Design review of the part built by this model. Coordinates are the model's own, in mm. A direction names the side the tool comes from. Coordinates: 2 decimals unless noted, no trailing zeros. Write each loop counter-clockwise with the first axis right and the second up, starting at its lowest first coordinate (ties: lowest second). Pieces come first, ordered by that corner, then holes. Notation, with made-up numbers: (86, 38.25) - (104, 38.25) arc R19 ccw to (104, 69.25) - close; hole circle Ø11 at (-21.5, -8.75). An arc over 180 degrees is marked (long way). One line per item, written item: value.
from build123d import *

# Parameters (mm, degrees)
F1_DEPTH = 30


with BuildPart() as f1:
    # F0 (on Front) → F1 (new body)
    with BuildSketch(Plane.XZ):
        with BuildLine():
            Line((-10.025, -10.025), (-10.025, -4.563699))
            Line((-10.025, -4.563699), (-8.201301, -2.74))
            Line((-8.201301, -2.74), (-8.125, -2.74))
            Line((-8.125, -2.74), (-8.125, -4.16967))
            Line((-8.125, -4.16967), (-7.125, -4.16967))
            Line((-7.125, -4.16967), (-6.125, -2.504835))
            Line((-6.125, -2.504835), (-6.125, -0.84))
            Line((-6.125, -0.84), (-9.129728, -0.84))
            Line((-9.129728, -0.84), (-12.025, -3.735272))
            Line((-12.025, -3.735272), (-16.854638, -12.46486))
            ThreePointArc((-16.854638, -12.46486), (-17.38041, -18.730472), (-12.025, -22.025))
            Line((-12.025, -22.025), (12.025, -22.025))
            ThreePointArc((12.025, -22.025), (17.29087, -18.900868), (17.072982, -12.781872))
            Line((17.072982, -12.781872), (12.025, -3.735272))
            Line((12.025, -3.735272), (9.129728, -0.84))
            Line((9.129728, -0.84), (6.125, -0.84))
            Line((6.125, -0.84), (6.125, -2.504835))
            Line((6.125, -2.504835), (7.125, -4.16967))
            Line((7.125, -4.16967), (8.125, -4.16967))
            Line((8.125, -4.16967), (8.125, -2.74))
            Line((8.125, -2.74), (8.201301, -2.74))
            Line((8.201301, -2.74), (10.025, -4.563699))
            Line((10.025, -4.563699), (10.025, -10.025))
            Line((10.025, -10.025), (4.636716, -10.025))
            Line((4.636716, -10.025), (2.811716, -8.2))
            Line((2.811716, -8.2), (-2.811716, -8.2))
            Line((-2.811716, -8.2), (-4.636716, -10.025))
            Line((-4.636716, -10.025), (-8.125, -10.025))
            Line((-8.125, -10.025), (-10.025, -10.025))
        make_face()
        with BuildLine():
            ThreePointArc((-14.436503, -19.21634), (-15.81745, -14.753261), (-12.025, -12.025))
            Line((-12.025, -12.025), (-1.797092, -12.025))
            Line((-1.797092, -12.025), (-1.245732, -12.853762))
            Line((-1.245732, -12.853762), (-10.966173, -19.320583))
            ThreePointArc((-10.966173, -19.320583), (-12.71795, -19.821483), (-14.436503, -19.21634))
        make_face(mode=Mode.SUBTRACT)
        with BuildLine():
            Line((4.803493, -20.025), (-4.803493, -20.025))
            Line((-4.803493, -20.025), (-1.661703, -17.934828))
            ThreePointArc((-1.661703, -17.934828), (0, -17.432575), (1.661703, -17.934828))
            Line((1.661703, -17.934828), (4.803493, -20.025))
        make_face(mode=Mode.SUBTRACT)
        with BuildLine():
            ThreePointArc((12.025, -12.025), (15.81745, -14.753261), (14.436503, -19.21634))
            ThreePointArc((14.436503, -19.21634), (12.71795, -19.821483), (10.966173, -19.320583))
            Line((10.966173, -19.320583), (1.245732, -12.853762))
            Line((1.245732, -12.853762), (1.797092, -12.025))
            Line((1.797092, -12.025), (12.025, -12.025))
        make_face(mode=Mode.SUBTRACT)
    extrude(amount=F1_DEPTH)


solid = f1.part
1. Consider section C-C, the plane x = 15. Write out the cut boundary in (y, z).
Answer block:
outline: (-30, -21.24) - (0, -21.24) - (0, -18.7) - (-30, -18.7) - close; (-30, -13.35) - (0, -13.35) - (0, -9.07) - (-30, -9.07) - close
2. Wall thickness on line 1 along Z through (x, y) = (-7, -19.5) (3 decimals); line 2 along X through (y, z) = (-6, -3.5) (3 decimals); line 3 along X through (y, z) = (-3.75, -8.5) (3 decimals): over which ranges is each line inside the solid? List them lowest first.
Answer block:
line 1: z = -22.025 to -16.682, -12.025 to -10.025, -3.962 to -0.84
line 2: x = -11.79 to -8.961, -8.125 to -6.723, 6.723 to 8.125, 8.961 to 11.79
line 3: x = -14.661 to -10.025, -3.112 to 3.112, 10.025 to 14.684
3. Insertion check: pin 1 Ø12 at (x, y) = (6, -6.5) entering from +Z; pin 2 Ø3 at (x, y) = (1, -20) entering from +Z; pin 3 Ø0.8 at (y, z) = (-13, -1.5) entering from +X; pin 4 Ø1.6 at (y, z) = (-9, -6.5) entering from -X. Each pin has a flat end and moves straight along its axis. Give the tip position at first contact, or say it passes through.
Answer block:
pin 1: stops at z = -0.84
pin 2: stops at z = -8.2
pin 3: stops at x = 10.19
pin 4: stops at x = -14
4. Consider section D-D, the plane z = -16.5. Write out the cut boundary in (x, y).
Answer block:
outline: (-18.01, -30) - (-16, -30) - (-16, 0) - (-18.01, 0) - close; (-6.73, -30) - (6.73, -30) - (6.73, 0) - (-6.73, 0) - close; (16, -30) - (18.01, -30) - (18.01, 0) - (16, 0) - close
5. Consider section B-B, the plane z = -6.75. Write out the cut boundary in (x, y) (3 decimals).
Answer block:
outline: (-13.693, -30) - (-10.025, -30) - (-10.025, 0) - (-13.693, 0) - close; (10.025, -30) - (13.707, -30) - (13.707, 0) - (10.025, 0) - close
6. Mouldability with a two-part tool opening along Z and no side actions: class faces 4 (the face through (14.584, -14.79, -8.322)), 5 (the face through (10.025, -15, -7)), 6 (the face through (-12.692, -14.79, -19.822)), 7 (the face through (-17.42, -14.79, -18.65)) as released by +Z, released by -Z, zero draft, split by the parting line, or undercut.
Answer block:
face 4: released by +Z
face 5: undercut
face 6: undercut
face 7: split by the parting line
7. For faces 1 (the face through (-10.56, -14.79, -2.27)), 2 (the face through (-7, -15, -10.025)), 3 (the face through (-6.125, -15, -2)), list the 3-axis set-ups (+Z, -Z, +X, -X, +Y, -Y) from which the entire face can be reached by the end or side of a thin tool; tool diameter is ignored.
Answer block:
face 1: +Z, -X, +Y, -Y
face 2: +Y, -Y
face 3: +Z, +Y, -Y
8. Consider section A-A, the plane x = -3.5. Write out the cut boundary in (y, z) (3 decimals).
Answer block:
outline: (-30, -22.025) - (0, -22.025) - (0, -20.025) - (-30, -20.025) - close; (-30, -19.158) - (0, -19.158) - (0, -14.353) - (-30, -14.353) - close; (-30, -12.025) - (0, -12.025) - (0, -8.888) - (-30, -8.888) - close
